Input: part model. Units: mm. Frame: model coordinates. A direction names the side the tool comes from. Round coordinates to 2 decimals unless told otherwise and drop trailing zeros. Loops run counter-clockwise (first coordinate to the right, second up) from the corner with the lowest first, then second, coordinate; pieces in that order, holes last.
1) Draft query along X for faces 5 (the face through (16.6, 62.07, 3.45)), 6 (the face through (12, 70, 3)), 7 (the face through (28, 9, 3)). Return one class per face: pulls with the +X half, pulls with the -X half, needs draft (parallel to the pull), parting line crosses it, or undercut.
2) Section C-C, the plane x = 24. Return loops of the section in (y, z).
3) First-contact query: pin 1 (6 mm diameter, centred on x = 32.5, z = 4, fed in from +Y); pin 2 (2.5 mm diameter, centred on x = -10.5, z = 1.5, fed in from +Y); pin 3 (8 mm diameter, centred on x = 28, y = 62.5, fed in from -Z). Flat tips, straight axial feed; report the tip coordinate or a pass-through.
4) Section D-D, the plane z = 26. Return loops of the section in (x, y), and give its area (3 significant figures).
5) Section B-B, the plane x = 17.25. Return loops of the section in (y, z), and give its area (3 significant figures).
6) Access query for faces 1 (the face through (33, 3, 9.5)), 2 (the face through (0, 40, 3)), 3 (the face through (34, 7, 4)), 4 (the face through (12, 41, 0)). Directions: +Z, -Z, +X, -X, +Y, -Y. A direction counts if a zero-diameter tool reaches every point of the face in a straight line with its end or side. Return the directions, or none.
7) Section A-A, the plane y = 65. Return loops of the section in (x, z).
8) Ray query, line 1 along Y through (x, z) = (17.25, 3.5); line 2 along Z through (x, y) = (17.5, 55); line 3 along Z through (x, y) = (-1, 3.5). Return the intervals inside material, ascending.
from build123d import *

# Parameters (mm, degrees)
SKETCH1_W           = 25
SKETCH1_H           = 70
SKETCH1_R           = 3
BOSS_EXTRUDE1_DEPTH = 7
SKETCH2_W           = 12
SKETCH2_H           = 24
SKETCH2_H_2         = 7
SKETCH2_W_2         = 6.5
SKETCH2_H_3         = 2.5
BOSS_EXTRUDE2_DEPTH = 7
CHAMFER2_SIZE       = 10
CHAMFER3_SIZE       = 5
CHAMFER4_SIZE       = 5
CHAMFER5_SIZE       = 2


with BuildPart() as part:
    # Sketch1 → Boss-Extrude1 (new body)
    with BuildSketch(Plane.XY):
        with Locations((12.5, 35)):
            Rectangle(SKETCH1_W, SKETCH1_H)
        with Locations((7.75, 65)):
            Circle(SKETCH1_R, mode=Mode.SUBTRACT)
        with Locations((17.25, 65)):
            Circle(SKETCH1_R, mode=Mode.SUBTRACT)
    extrude(amount=BOSS_EXTRUDE1_DEPTH)

    # Sketch2 → Boss-Extrude2 (add)
    with BuildSketch(Plane.XZ):
        with Locations((12.5, 21.5)):
            Rectangle(SKETCH2_W, SKETCH2_H)
        Polygon((6.5, 7), (6.5, 9.5), (-12.5, 9.5), (-12.5, -2.5), (6.5, -2.5), (6.5, 0), (0, 0), (0, 7), align=None)
        with Locations((12.5, 3.5)):
            Rectangle(SKETCH2_W, SKETCH2_H_2)
        Polygon((37.5, 9.5), (18.5, 9.5), (18.5, 7), (25, 7), (25, 0), (18.5, 0), (18.5, -2.5), (37.5, -2.5), align=None)
        with Locations((12.5, -14.5)):
            Rectangle(SKETCH2_W, SKETCH2_H)
        with Locations((3.25, 3.5)):
            Rectangle(SKETCH2_W_2, SKETCH2_H_2)
        with Locations((12.5, 8.25)):
            Rectangle(SKETCH2_W, SKETCH2_H_3)
        with Locations((12.5, -1.25)):
            Rectangle(SKETCH2_W, SKETCH2_H_3)
        with Locations((21.75, 3.5)):
            Rectangle(SKETCH2_W_2, SKETCH2_H_2)
    extrude(amount=-BOSS_EXTRUDE2_DEPTH)

    # Chamfer2
    chamfer2_edges = [part.edges().sort_by_distance(p)[0] for p in [
        (18.5, 3.5, 9.5),
        (18.5, 3.5, -2.5),
        (6.5, 3.5, -2.5),
        (6.5, 3.5, 9.5),
    ]]
    chamfer(chamfer2_edges, length=CHAMFER2_SIZE)

    # Chamfer3
    chamfer3_edges = [part.edges().sort_by_distance(p)[0] for p in [
        (12.5, 7, 7),
        (12.5, 7, 0),
    ]]
    chamfer(chamfer3_edges, length=CHAMFER3_SIZE)

    # Chamfer4
    # the kernel refuses this chamfer: 5 mm, written as the material it adds along each edge
    with BuildSketch(Plane(origin=(25, 7, -17.85841494), x_dir=(0.9996219169112968, -0.027495876610586317, 0), z_dir=(0, 0, 1))) as chamfer4_piece_1_section:
        Polygon((CHAMFER4_SIZE * 0.999621916911, CHAMFER4_SIZE * 0.0274958766106), (-CHAMFER4_SIZE * 0.0274958766106, CHAMFER4_SIZE * 0.999621916911), (0, 0), align=None)
    chamfer4_piece_1 = extrude(amount=42.71682988, mode=Mode.PRIVATE)
    chamfer4_piece_1 = split(chamfer4_piece_1, bisect_by=Plane(origin=(26.380997475, 7.88604798, 9.5), z_dir=(0, 0, -1)), keep=Keep.TOP, mode=Mode.PRIVATE)
    chamfer4_piece_1 = split(chamfer4_piece_1, bisect_by=Plane(origin=(27.086016414, 7.88604798, -3.913983586), z_dir=(-0.7071067811865475, 0, 0.7071067811865477)), keep=Keep.TOP, mode=Mode.PRIVATE)
    chamfer4_piece_1 = split(chamfer4_piece_1, bisect_by=Plane(origin=(26.380997475, 8.338541667, -3.661458333), z_dir=(0, -0.7071067811865476, 0.7071067811865476)), keep=Keep.TOP, mode=Mode.PRIVATE)
    chamfer4_piece_1 = split(chamfer4_piece_1, bisect_by=Plane(origin=(26.380997475, 15.047506313, 3.952493687), z_dir=(0, -0.7071067811865476, -0.7071067811865476)), keep=Keep.TOP, mode=Mode.PRIVATE)
    add(chamfer4_piece_1)
    with BuildSketch(Plane(origin=(25, 7, -17.85841494), x_dir=(0.9996219169112968, -0.027495876610586317, 0), z_dir=(0, 0, 1))) as chamfer4_piece_2_section:
        Polygon((CHAMFER4_SIZE * 0.999621916911, CHAMFER4_SIZE * 0.0274958766106), (-CHAMFER4_SIZE * 0.0274958766106, CHAMFER4_SIZE * 0.999621916911), (0, 0), align=None)
    chamfer4_piece_2 = extrude(amount=42.71682988, mode=Mode.PRIVATE)
    chamfer4_piece_2 = split(chamfer4_piece_2, bisect_by=Plane(origin=(34.6875, 7.375, 3.3125), z_dir=(-0.7071067811865475, 0, -0.7071067811865477)), keep=Keep.TOP, mode=Mode.PRIVATE)
    chamfer4_piece_2 = split(chamfer4_piece_2, bisect_by=Plane(origin=(29.25, 7.375, -2.5), z_dir=(0, 0, 1)), keep=Keep.TOP, mode=Mode.PRIVATE)
    chamfer4_piece_2 = split(chamfer4_piece_2, bisect_by=Plane(origin=(29.25, 8.625, -3.375), z_dir=(0, -0.7071067811865476, 0.7071067811865476)), keep=Keep.TOP, mode=Mode.PRIVATE)
    chamfer4_piece_2 = split(chamfer4_piece_2, bisect_by=Plane(origin=(29.25, 14.25, 4.75), z_dir=(0, -0.7071067811865476, -0.7071067811865476)), keep=Keep.TOP, mode=Mode.PRIVATE)
    add(chamfer4_piece_2)
    with BuildSketch(Plane(origin=(0, 7, 24.85841494), x_dir=(-0.9996219169112968, -0.027495876610586317, 0), z_dir=(0, 0, -1))) as chamfer4_piece_3_section:
        Polygon((CHAMFER4_SIZE * 0.999621916911, CHAMFER4_SIZE * 0.0274958766106), (-CHAMFER4_SIZE * 0.0274958766106, CHAMFER4_SIZE * 0.999621916911), (0, 0), align=None)
    chamfer4_piece_3 = extrude(amount=42.71682988, mode=Mode.PRIVATE)
    chamfer4_piece_3 = split(chamfer4_piece_3, bisect_by=Plane(origin=(-2.086016414, 7.88604798, 10.913983586), z_dir=(0.7071067811865477, 0, -0.7071067811865475)), keep=Keep.TOP, mode=Mode.PRIVATE)
    chamfer4_piece_3 = split(chamfer4_piece_3, bisect_by=Plane(origin=(-1.380997475, 7.88604798, -2.5), z_dir=(0, 0, 1)), keep=Keep.TOP, mode=Mode.PRIVATE)
    chamfer4_piece_3 = split(chamfer4_piece_3, bisect_by=Plane(origin=(-1.380997475, 15.047506313, 3.047506313), z_dir=(0, -0.7071067811865476, 0.7071067811865476)), keep=Keep.TOP, mode=Mode.PRIVATE)
    chamfer4_piece_3 = split(chamfer4_piece_3, bisect_by=Plane(origin=(-1.380997475, 8.338541667, 10.661458333), z_dir=(0, -0.7071067811865476, -0.7071067811865476)), keep=Keep.TOP, mode=Mode.PRIVATE)
    add(chamfer4_piece_3)
    with BuildSketch(Plane(origin=(0, 7, 24.85841494), x_dir=(-0.9996219169112968, -0.027495876610586317, 0), z_dir=(0, 0, -1))) as chamfer4_piece_4_section:
        Polygon((CHAMFER4_SIZE * 0.999621916911, CHAMFER4_SIZE * 0.0274958766106), (-CHAMFER4_SIZE * 0.0274958766106, CHAMFER4_SIZE * 0.999621916911), (0, 0), align=None)
    chamfer4_piece_4 = extrude(amount=42.71682988, mode=Mode.PRIVATE)
    chamfer4_piece_4 = split(chamfer4_piece_4, bisect_by=Plane(origin=(-4.25, 7.375, 9.5), z_dir=(0, 0, -1)), keep=Keep.TOP, mode=Mode.PRIVATE)
    chamfer4_piece_4 = split(chamfer4_piece_4, bisect_by=Plane(origin=(-9.6875, 7.375, 3.6875), z_dir=(0.7071067811865476, 0, 0.7071067811865475)), keep=Keep.TOP, mode=Mode.PRIVATE)
    chamfer4_piece_4 = split(chamfer4_piece_4, bisect_by=Plane(origin=(-4.25, 14.25, 2.25), z_dir=(0, -0.7071067811865476, 0.7071067811865476)), keep=Keep.TOP, mode=Mode.PRIVATE)
    chamfer4_piece_4 = split(chamfer4_piece_4, bisect_by=Plane(origin=(-4.25, 8.625, 10.375), z_dir=(0, -0.7071067811865476, -0.7071067811865476)), keep=Keep.TOP, mode=Mode.PRIVATE)
    add(chamfer4_piece_4)

    # Chamfer5
    chamfer5_edges = [part.edges().sort_by_distance(p)[0] for p in [
        (0, 70, 3.5),
        (25, 70, 3.5),
    ]]
    chamfer(chamfer5_edges, length=CHAMFER5_SIZE)


solid = part.part
Final values:
1. face 5: undercut
1. face 6: needs draft
1. face 7: pulls with the +X half
2. outline: (0, -7) - (7, -7) - (7, -5) - (12, 0) - (69, 0) - (69, 7) - (12, 7) - (7, 12) - (7, 14) - (0, 14) - close
3. pin 1: stops at y = 7.5
3. pin 2: stops at y = 7
3. pin 3: stops at z = 0
4. outline: (6.5, 0) - (18.5, 0) - (18.5, 7) - (6.5, 7) - close
4. area: 84.0 mm2
5. outline: (0, -26.5) - (7, -26.5) - (7, -5) - (12, 0) - (62, 0) - (62, 7) - (12, 7) - (7, 12) - (7, 33.5) - (0, 33.5) - close; (68, 0) - (70, 0) - (70, 7) - (68, 7) - close
5. area: 844 mm2
6. face 1: +Z, +X, +Y, -Y
6. face 2: +Z, -Z, -X, +Y
6. face 3: +Z, -Z, +X, +Y
6. face 4: -Z, +X, -X, +Y
7. outline: (0, 0) - (4.75, 0) - (4.75, 7) - (0, 7) - close; (10.75, 0) - (14.25, 0) - (14.25, 7) - (10.75, 7) - close; (20.25, 0) - (25, 0) - (25, 7) - (20.25, 7) - close
8. line 1: y = 0 to 62, 68 to 70
8. line 2: z = 0 to 7
8. line 3: z = -5 to 12
